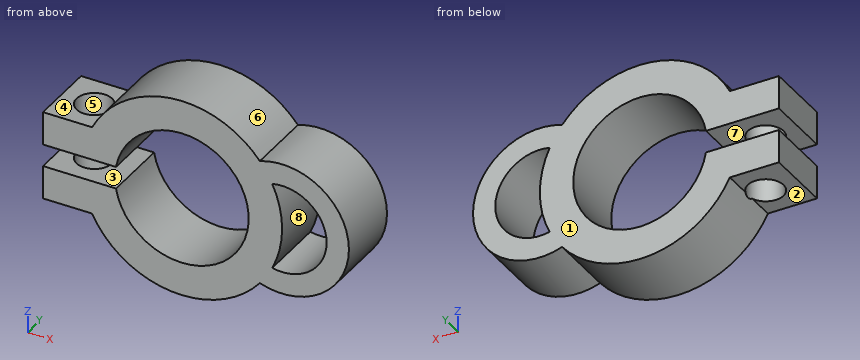
Autodesk Inventor part; units mm, degrees
ref_plane "YZ Plane" through (0, 0, 0) normal (1, 0, 0) x (0, 1, 0)
ref_plane "XZ Plane" through (0, 0, 0) normal (0, 1, 0) x (-1, 0, 0)
ref_plane "XY Plane" through (0, 0, 0) normal (0, 0, 1) x (1, 0, 0)
sketch "Sketch1" plane through (0, 0, 0) normal (0, 1, 0) x (-1, 0, 0)
  circle A0 centre (0, 0) radius 6
  circle A1 centre (0, 0) radius 9
  line L0 (4.4721, 4) -> (12.4721, 4)
  line L1 (12.4721, 4) -> (12.4721, 1)
  line L2 (12.4721, 1) -> (4.4721, 1)
  line L3 (4.4721, 1) -> (4.4721, 4)
  line L4 (4.4721, -4) -> (12.4721, -4)
  line L5 (12.4721, -4) -> (12.4721, -1)
  line L6 (12.4721, -1) -> (4.4721, -1)
  line L7 (4.4721, -1) -> (4.4721, -4)
  circle A2 centre (-9, 0) radius 4
  circle A3 centre (-9, 0) radius 6
  point P0 (-8.1111, -3.9)
  point P1 (-8.1111, 3.9)
  point P2 (5.9161, 1)
  point P3 (8.0623, 4)
  point P4 (-7, 5.6569)
  point P5 (-7, -5.6569)
  point P6 (8.0623, -4)
  point P7 (5.9161, -1)
  dimension "d0" = 12
  dimension "d1" = 3
  dimension "d2" = 3
  dimension "d3" = 3
  dimension "d4" = 1
  dimension "d5" = 1
  dimension "d6" = 8
  dimension "d7" = 8
  dimension "d8" = 8
  dimension "d9" = 2
extrude "Extrusion1" add sketch "Sketch1" along normal blind 6 contours A0 L0 A1 L2 | L6 A1 L4 A0 | A0 A3 A1 L0 | A1 L0 L1 L2 | L4 A1 A3 A0 | L6 L5 L4 A1 | A0 A2 A1 A3 | A3 A1 A2 A0 | A0 A2 A1 | A1 A2 A3
sketch "Sketch2" plane through (-12.4721, 0, 4) normal (0, 0, 1) x (1, 0, 0)
  line L0 (0, 0) -> (4.4099, 0)
  line L1 (4.4099, 0) -> (4.4099, 6)
  line L2 (0, 6) -> (4.4099, 6)
  line L3 (0, 0) -> (0, 6)
  circle A0 centre (2.8989, 3) radius 1.6
  point P0 (12.4721, 0)
  dimension "d12" = 3.2
extrude "Extrusion2" cut sketch "Sketch2" against normal blind 10 contours A0 L1 | L1 A0
properties part number "Spring_hook"
Could you check a few things on this model? Use its own coordinates, in mm. Face numbers are marked on the shaded views. A direction names the side the tool comes from. Give positions to 0.01 mm unless a question says otherwise; leave off trailing zeros. Loops run counter-clockwise (first coordinate to the right, second up) from the corner with the lowest first, then second, coordinate; pieces in that order, holes last. Notation, with made-up numbers: M 61.25,22.5 L 80.25,22.5 A27 ccw 80.25,49.5 Z; hole C 70,87.25 d9. An arc over 180 degrees is marked long. Answer as a JSON object with one key per item and string values.
Q1. For the marked faces 1, 2, 3 and 4, which set-ups out of +Z, -Z, +X, -X, +Y, -Y let a thin tool reach every point of the face, with its end or its side?
Values found:
{"face 1": "+Z, -Z, +X, -X, +Y", "face 2": "-Z, -X, +Y, -Y", "face 3": "-X, +Y, -Y", "face 4": "+Z, -X, +Y, -Y"}
Q2. Suppose I cut it at A-A, the plane x = 0. List the corners of the cut face in (y, z) for me.
Values found:
{"outline": "M 0,-9 L 6,-9 L 6,-6 L 0,-6 Z; M 0,6 L 6,6 L 6,9 L 0,9 Z"}
Q3. Suppose I cut it at B-B, the plane z = 0. List the corners of the cut face in (x, y) for me, plus the area to 3 significant figures.
Values found:
{"outline": "M 6,0 L 9,0 L 9,6 L 6,6 Z; M 13,0 L 15,0 L 15,6 L 13,6 Z", "area": "30.0 mm²"}
Q4. If we mould it in two halves opening along Z, with no side actions, what happens to the marked faces 5, 6, 7 and 8? For each: pulls with the +Z half, pulls with the -Z half, needs draft (parallel to the pull), parting line crosses it, or undercut.
Values found:
{"face 5": "needs draft", "face 6": "pulls with the +Z half", "face 7": "undercut", "face 8": "undercut"}
Q5. For P1, Ø3, axis at x = -5, y = 1, coming from the +Z side; P2, Ø1, axis at x = -6.5, y = 1.5, coming from the -Z side; P3, Ø3, axis at x = -9.5, y = 4, coming from the +Z side, each with a flat end and sliding along its axis, tell me the tip position at first contact or that it passes through.
Values found:
{"P1": "stops at z = 8.29", "P2": "stops at z = -6.71", "P3": "stops at z = 4.12"}
Q6. Suppose I cut it at D-D, the plane z = 2.5. List the corners of the cut face in (x, y) for me, plus the area to 3 significant figures.
Values found:
{"outline": "M -12.47,0 L -5.45,0 L -5.45,6 L -12.47,6 Z; M 5.45,0 L 8.65,0 L 8.65,6 L 5.45,6 Z; M 12.12,0 L 14.45,0 L 14.45,6 L 12.12,6 Z; hole C -9.57,3 d3.2", "area": "67.2 mm²"}
Q7. If I drill on probe 1 along X at (y, z) = (5.75, 2.5); probe 2 along Z at (x, y) = (3.25, 5.75); probe 3 along Z at (x, y) = (0, 3), over which ranges is the centre line in solid material (lowest first)? Write a range as [from, to].
Values found:
{"probe 1": "x = [-12.47, -5.45], [5.45, 8.65], [12.12, 14.45]", "probe 2": "z = [-8.39, -5.04], [5.04, 8.39]", "probe 3": "z = [-9, -6], [6, 9]"}
Q8. Suppose I cut it at C-C, the plane y = 5.5. List the corners of the cut face in (x, z) for me, plus the area to 3 significant figures.
Values found:
{"outline": "M -12.47,-4 L -8.06,-4 A9 ccw 7,-5.66 A6 ccw long 7,5.66 A9 ccw -8.06,4 L -12.47,4 L -12.47,1 L -5.92,1 A6 cw long -5.92,-1 L -12.47,-1 Z; hole M 8.11,-3.9 A4 ccw long 8.11,3.9 A9 cw Z", "area": "196 mm²"}
